Part model, mm, in its own coordinate system. A direction names the side the tool comes from. Round coordinates to 2 decimals unless told otherwise and drop trailing zeros. Loops run counter-clockwise (first coordinate to the right, second up) from the corner with the lowest first, then second, coordinate; pieces in that order, holes last. Notation, with made-up numbers: M -22,-30.5 L -6,-30.5 A9 cw -6,-23.5 Z; hole C 69,-17 d10. An arc over 180 degrees is marked long. Put each result on its own line as item: value. Start each with the question number.
1) Pull direction Z, two halves, no side cores. Call faces 1 (the flat face through (-7.5, 28, -37)), 2 (the cylindrical face through (-60.72, 27.83, -0.88)), 3 (the cylindrical face through (-56.044, 38.028, -0.221)): +Z half, -Z half, draft (parallel to the pull), parting line (faces both ways), or undercut.
2) Slice it at C-C on x = -13. Give the cut face in (y, z).
3) Which spindle directions (+Z, -Z, +X, -X, +Y, -Y) get a long thin tool onto all of the face, cutting with end or side? Do faces 4 (the flat face through (12, 7, -22.348)), 5 (the flat face through (11, 5, 60)), 6 (the flat face through (-20, 20, 37)), 7 (the flat face through (11, 10, 48)). Say none if no direction does.
4) Slice it at A-A on x = 38. Give the cut face in (y, z), then the cut area to 3 significant figures.
5) Drop flat-ended pins along their axis: pin 1 Ø6 at (x, y) = (50.5, 24.5) entering from -Z; pin 2 Ø1.5 at (x, y) = (34, 18.5) entering from -Z; pin 3 Ø4 at (x, z) = (54.345, -44.68) entering from +Y; pin 4 Ø8.5 at (x, z) = (54.345, -44.68) entering from +Y. Give the stop position or say it passes through.
6) Slice it at B-B on y = 30. Give the cut face in (x, z), then the cut area to 3 significant figures.
7) Probe line 1 along X through (y, z) = (8.5, -45) (3 decimals); line 2 along X through (y, z) = (8.6, -91) (3 decimals); line 3 along Y through (x, z) = (58.5, 13.5). List the from-to ranges inside material, lowest first.
```python
from build123d import *

# Parameters (mm, degrees)
BOSS_EXTRUDE1_DEPTH     = 10
BOSS_EXTRUDE2_START     = 10
BOSS_EXTRUDE2_DEPTH     = 30
SKETCH8_W               = 150
SKETCH8_H               = 154
BOSS_EXTRUDE3_DEPTH     = 10
CUT_EXTRUDE2_START      = 10
SKETCH5_R               = 11.15
CUT_EXTRUDE2_DEPTH      = 7.5
CUT_EXTRUDE4_DEPTH      = 135.270280498
CUT_EXTRUDE4_DEPTH_BACK = 135.270280498
SKETCH7_W               = 25
SKETCH7_H               = 16
CHAMFER1_SIZE           = 6
FILLET1_R               = 25
CUT_EXTRUDE5_START      = 40
SKETCH9_R               = 1.5
SKETCH9_R_2             = 1.7
CUT_EXTRUDE5_DEPTH      = 4
CUT_EXTRUDE6_DEPTH      = 176.297069285
CUT_EXTRUDE6_DEPTH_BACK = 176.297069285
SKETCH10_R              = 1.45
CUT_EXTRUDE7_DEPTH      = 135.270280563
CUT_EXTRUDE7_DEPTH_BACK = 4
CUT_EXTRUDE7_START      = 10
SKETCH11_R              = 3.25
CUT_EXTRUDE8_START      = 10
CUT_EXTRUDE8_DEPTH      = 6


with BuildPart() as part:
    # Sketch1 → Boss-Extrude1 (new body)
    with BuildSketch(Plane(origin=(0, 0, 0), x_dir=(1, 0, 0), z_dir=(0, 1, 0))):
        with BuildLine():
            Line((45, 40), (-20.73, 40))
            ThreePointArc((-20.73, 40), (-60.73, 0), (-20.73, -40))
            Line((-20.73, -40), (45, -40))
            ThreePointArc((45, -40), (85, 0), (45, 40))
        make_face()
    extrude(amount=BOSS_EXTRUDE1_DEPTH)

    # Sketch2 → Boss-Extrude2 (add)
    with BuildSketch(Plane(origin=(0, 0, 0), x_dir=(1, 0, 0), z_dir=(0, 1, 0)).offset(BOSS_EXTRUDE2_START)):
        with BuildLine():
            Line((-20.73, -40), (45, -40))
            ThreePointArc((45, -40), (85, 0), (45, 40))
            Line((45, 40), (-20.73, 40))
            ThreePointArc((-20.73, 40), (-60.73, 0), (-20.73, -40))
        make_face()
        with BuildLine():
            Line((45, 34), (-20.73, 34))
            ThreePointArc((-20.73, 34), (-54.73, 0), (-20.73, -34))
            Line((-20.73, -34), (45, -34))
            ThreePointArc((45, -34), (79, 0), (45, 34))
        make_face(mode=Mode.SUBTRACT)
    extrude(amount=BOSS_EXTRUDE2_DEPTH)

    # Sketch8 → Boss-Extrude3 (add)
    with BuildSketch(Plane(origin=(0, 0, 0), x_dir=(1, 0, 0), z_dir=(0, 1, 0))):
        with Locations((12.135, 17)):
            Rectangle(SKETCH8_W, SKETCH8_H)
    extrude(amount=BOSS_EXTRUDE3_DEPTH)

    # Sketch5 → Cut-Extrude2 (cut)
    with BuildSketch(Plane(origin=(0, 0, 0), x_dir=(1, 0, 0), z_dir=(0, 1, 0)).offset(CUT_EXTRUDE2_START)):
        with Locations(Location((-20.73, 0, 0), (0, 0, 270))):
            Circle(SKETCH5_R)
        with Locations(Location((38, 0, 0), (0, 0, 270))):
            Circle(SKETCH5_R)
    extrude(amount=-CUT_EXTRUDE2_DEPTH, mode=Mode.SUBTRACT)

    # Sketch7 → Cut-Extrude4 (cut, two sides: drawn at the far end of the back side and taken through both)
    with BuildSketch(Plane.XY.offset(-CUT_EXTRUDE4_DEPTH_BACK)):
        with Locations((-20, 28)):
            Rectangle(SKETCH7_W, SKETCH7_H)
        with Locations((45, 28)):
            Rectangle(SKETCH7_W, SKETCH7_H)
    extrude(amount=CUT_EXTRUDE4_DEPTH + CUT_EXTRUDE4_DEPTH_BACK, mode=Mode.SUBTRACT)

    # Chamfer1
    # the kernel refuses this chamfer: 6 mm, written as the material it adds along each edge
    with BuildSketch(Plane(origin=(-20.73, 10, 40), x_dir=(0, 0.9996219169112968, -0.02749587661058678), z_dir=(1, 0, 0))) as chamfer1_piece_1:
        Polygon((CHAMFER1_SIZE * 0.999621916911, CHAMFER1_SIZE * 0.0274958766106), (-CHAMFER1_SIZE * 0.0274958766106, CHAMFER1_SIZE * 0.999621916911), (0, 0), align=None)
    extrude(amount=65.73)
    with BuildSketch(Plane(origin=(45, 10, -40), x_dir=(0, -0.02749587661058648, -0.9996219169112968), z_dir=(-1, 0, 0))) as chamfer1_piece_2:
        Polygon((CHAMFER1_SIZE * 0.999621916911, -CHAMFER1_SIZE * 0.0274958766106), (-CHAMFER1_SIZE * 0.0274958766106, -CHAMFER1_SIZE * 0.999621916911), (0, 0), align=None)
    extrude(amount=65.73)
    with BuildSketch(Plane(origin=(45, 10, 0), x_dir=(0, 0, -1), z_dir=(-1, 0, 0))) as chamfer1_piece_3_section:
        Polygon((40 + CHAMFER1_SIZE, 0), (40, -CHAMFER1_SIZE), (40, 0), align=None)
    chamfer1_piece_3 = revolve(axis=Axis((45, 10, 0), (0, -1, 0)), revolution_arc=180, mode=Mode.PRIVATE)
    chamfer1_piece_3 = split(chamfer1_piece_3, bisect_by=Plane(origin=(87.135, 10.791585947, -38.986610485), z_dir=(-1, 0, 0)), keep=Keep.TOP, mode=Mode.PRIVATE)
    add(chamfer1_piece_3)
    with BuildSketch(Plane(origin=(-20.73, 10, 0), x_dir=(0, 0, 1), z_dir=(1, 0, 0))) as chamfer1_piece_4_section:
        Polygon((40, -CHAMFER1_SIZE), (40 + CHAMFER1_SIZE, 0), (40, 0), align=None)
    chamfer1_piece_4 = revolve(axis=Axis((-20.73, 10, 0), (0, -1, 0)), revolution_arc=180, mode=Mode.PRIVATE)
    chamfer1_piece_4 = split(chamfer1_piece_4, bisect_by=Plane(origin=(-62.865, 15.017860126, 35.326549698), z_dir=(1, 0, 0)), keep=Keep.TOP, mode=Mode.PRIVATE)
    add(chamfer1_piece_4)

    # Fillet1
    fillet1_edges = [part.edges().sort_by_distance(p)[0] for p in [
        (87.135, 5, 60),
        (87.135, 5, -94),
        (-62.865, 5, -94),
        (-62.865, 5, 60),
    ]]
    fillet(fillet1_edges, radius=FILLET1_R)

    # Sketch9 → Cut-Extrude5 (cut)
    with BuildSketch(Plane(origin=(0, 0, 0), x_dir=(1, 0, 0), z_dir=(0, 1, 0)).offset(CUT_EXTRUDE5_START)):
        with Locations(Location((45, -37, 0), (0, 0, 270))):
            Circle(SKETCH9_R)
        with Locations(Location((-20.73, -37, 0), (0, 0, 270))):
            Circle(SKETCH9_R)
        with Locations(Location((45, 37, 0), (0, 0, 270))):
            Circle(SKETCH9_R)
        with Locations(Location((-20.73, 37, 0), (0, 0, 270))):
            Circle(SKETCH9_R)
        with Locations(Location((-57.73, 0, 0), (0, 0, 270))):
            Circle(SKETCH9_R_2)
        with Locations(Location((82, 0, 0), (0, 0, 270))):
            Circle(SKETCH9_R_2)
    extrude(amount=-CUT_EXTRUDE5_DEPTH, mode=Mode.SUBTRACT)

    # Sketch10 → Cut-Extrude6 (cut, two sides: drawn at the far end of the back side and taken through both)
    with BuildSketch(Plane(origin=(-45.015, 10, -51.2), x_dir=(1, 0, 0), z_dir=(0, 1, 0)).offset(-CUT_EXTRUDE6_DEPTH_BACK)):
        with Locations(Location((14.94, -6.52, 0), (0, 0, 270))):
            Circle(SKETCH10_R)
        with Locations(Location((99.36, -6.52, 0), (0, 0, 270))):
            Circle(SKETCH10_R)
        with Locations(Location((99.36, 39.8, 0), (0, 0, 270))):
            Circle(SKETCH10_R)
        with Locations(Location((14.94, 39.8, 0), (0, 0, 270))):
            Circle(SKETCH10_R)
    extrude(amount=CUT_EXTRUDE6_DEPTH + CUT_EXTRUDE6_DEPTH_BACK, mode=Mode.SUBTRACT)

    # Sketch11 → Cut-Extrude7 (cut, two sides: drawn at the far end of the back side and taken through both)
    with BuildSketch(Plane(origin=(0, 0, 0), x_dir=(1, 0, 0), z_dir=(0, 1, 0)).offset(CUT_EXTRUDE7_START - CUT_EXTRUDE7_DEPTH_BACK)):
        with Locations(Location((-30.075, 44.68, 0), (0, 0, 90))):
            Circle(SKETCH11_R)
        with Locations((-30.075, 91)):
            Circle(SKETCH11_R)
        with Locations((54.345, 91)):
            Circle(SKETCH11_R)
        with Locations(Location((54.345, 44.68, 0), (0, 0, 90))):
            Circle(SKETCH11_R)
    extrude(amount=CUT_EXTRUDE7_DEPTH + CUT_EXTRUDE7_DEPTH_BACK, mode=Mode.SUBTRACT)

    # Sketch12 → Cut-Extrude8 (cut)
    with BuildSketch(Plane(origin=(0, 0, 0), x_dir=(1, 0, 0), z_dir=(0, 1, 0)).offset(CUT_EXTRUDE8_START)):
        with BuildLine():
            Line((15.135, 22.347672995), (9.135, 22.347672995))
            ThreePointArc((9.135, 22.347672995), (7.720786438, 21.761886557), (7.135, 20.347672995))
            Line((7.135, 20.347672995), (7.135, -15.652327005))
            ThreePointArc((7.135, -15.652327005), (7.720786438, -17.066540567), (9.135, -17.652327005))
            Line((9.135, -17.652327005), (15.135, -17.652327005))
            ThreePointArc((15.135, -17.652327005), (16.549213562, -17.066540567), (17.135, -15.652327005))
            Line((17.135, -15.652327005), (17.135, 20.347672995))
            ThreePointArc((17.135, 20.347672995), (16.549213562, 21.761886557), (15.135, 22.347672995))
        make_face()
    extrude(amount=-CUT_EXTRUDE8_DEPTH, mode=Mode.SUBTRACT)


solid = part.part
```
Recorded:
1. face 1: draft
1. face 2: parting line
1. face 3: undercut
2. outline: M 0,-94 L 10,-94 L 10,-46 L 16,-40 L 20,-40 L 20,-34 L 10,-34 L 10,-8.04 L 2.5,-8.04 L 2.5,8.04 L 10,8.04 L 10,34 L 20,34 L 20,40 L 16,40 L 10,46 L 10,60 L 0,60 Z; M 36,-40 L 40,-40 L 40,-34 L 36,-34 Z; M 36,34 L 40,34 L 40,40 L 36,40 Z
3. face 4: +Y
3. face 5: +Z, +X, -X, +Y, -Y
3. face 6: +Z, -Z
3. face 7: +Z, +Y
4. outline: M 0,-94 L 10,-94 L 10,-46 L 16,-40 L 20,-40 L 20,-34 L 10,-34 L 10,-11.15 L 2.5,-11.15 L 2.5,11.15 L 10,11.15 L 10,34 L 20,34 L 20,40 L 16,40 L 10,46 L 10,60 L 0,60 Z; M 36,-40 L 40,-40 L 40,-34 L 36,-34 Z; M 36,34 L 40,34 L 40,40 L 36,40 Z
4. area: 1,580 mm2
5. pin 1: passes through
5. pin 2: stops at z = -40
5. pin 3: stops at y = 6
5. pin 4: stops at y = 14.6
6. outline: M -32.5,-38.23 L -32.5,-31.9 A34 cw -32.5,31.9 L -32.5,38.23 A40 ccw Z; M -7.5,-40 L 32.5,-40 L 32.5,-34 L -7.5,-34 Z; M -7.5,34 L 32.5,34 L 32.5,40 L -7.5,40 Z; M 57.5,-38 A40 ccw 57.5,38 L 57.5,31.62 A34 cw 57.5,-31.62 Z
6. area: 1,580 mm2
7. line 1: x = -62.865 to -33.309, -26.841 to 51.111, 57.579 to 87.135
7. line 2: x = -49.739 to -33.325, -26.825 to 51.095, 57.595 to 74.009
7. line 3: y = 0 to 10
